```python
from build123d import *

# Parameters (mm, degrees)
ESQUISSE1_W                  = 70
ESQUISSE1_H                  = 25
BOSS_EXTRU_1_DEPTH           = 25
ENL_V_MAT_EXTRU_1_DEPTH      = 79.421935707
ENL_V_MAT_EXTRU_1_DEPTH_BACK = 79.421935707
CONG_1_R                     = 5
CONG_2_R                     = 2
ENL_V_MAT_EXTRU_2_DEPTH      = 79.421935739
ENL_V_MAT_EXTRU_2_DEPTH_BACK = 79.421935739
ESQUISSE3_R                  = 8


with BuildPart() as part:
    # Esquisse1 → Boss.-Extru.1 (new body)
    with BuildSketch(Plane.XY):
        with Locations((35, 12.5)):
            Rectangle(ESQUISSE1_W, ESQUISSE1_H)
    extrude(amount=BOSS_EXTRU_1_DEPTH)

    # Esquisse2 → Enlèv. mat.-Extru.1 (cut, two sides: drawn at the far end of the back side and taken through both)
    with BuildSketch(Plane.XY.offset(25).offset(-ENL_V_MAT_EXTRU_1_DEPTH_BACK)):
        with BuildLine():
            Line((30, 25), (0, 25))
            Line((0, 25), (0, 10))
            ThreePointArc((0, 10), (16.648162051, 14.203675898), (30, 25))
        make_face()
    extrude(amount=ENL_V_MAT_EXTRU_1_DEPTH + ENL_V_MAT_EXTRU_1_DEPTH_BACK, mode=Mode.SUBTRACT)

    # Congé1
    cong_1_edges = [part.edges().sort_by_distance(p)[0] for p in [
        (30, 25, 12.5),
        (0, 10, 12.5),
        (70, 25, 12.5),
        (70, 0, 12.5),
        (0, 0, 12.5),
    ]]
    fillet(cong_1_edges, radius=CONG_1_R)

    # Congé2
    cong_2_edges = [part.edges().sort_by_distance(p)[0] for p in [
        (35, 0, 0),
        (35, 0, 25),
        (17.598161914, 14.694657605, 0),
        (48.658916792, 25, 0),
        (70, 12.5, 0),
        (0, 5.207778491, 0),
        (68.535533906, 23.535533906, 0),
        (68.535533906, 1.464466094, 0),
        (1.227276928, 8.696800743, 0),
        (30.275283676, 24.563769261, 0),
        (1.464466094, 1.464466094, 0),
        (0, 5.207778491, 25),
        (48.658916792, 25, 25),
        (17.598161914, 14.694657605, 25),
        (70, 12.5, 25),
        (68.535533906, 23.535533906, 25),
        (68.535533906, 1.464466094, 25),
        (1.227276928, 8.696800743, 25),
        (30.275283676, 24.563769261, 25),
        (1.464466094, 1.464466094, 25),
    ]]
    fillet(cong_2_edges, radius=CONG_2_R)

    # Esquisse3 → Enlèv. mat.-Extru.2 (cut, two sides: drawn at the far end of the back side and taken through both)
    with BuildSketch(Plane(origin=(0, 25, 0), x_dir=(1, 0, 0), z_dir=(0, 1, 0)).offset(-ENL_V_MAT_EXTRU_2_DEPTH_BACK)):
        with Locations(Location((45, -12.5, 0), (0, 0, 270))):
            Circle(ESQUISSE3_R)
    extrude(amount=ENL_V_MAT_EXTRU_2_DEPTH + ENL_V_MAT_EXTRU_2_DEPTH_BACK, mode=Mode.SUBTRACT)


solid = part.part
```
Can you work these out from the model? Positions are in its coordinate system, mm. Give positions to 0.01 mm unless a question says otherwise; leave off trailing zeros. Order: outer loops, then holes, each group sorted by start corner. A loop starts at its lowest first (then second) coordinate and runs counter-clockwise, first axis right, second up. Notation, with made-up numbers: (31.25, 57) - (66.25, 57) arc R14 ccw to (66.25, 68) - close; hole circle Ø5 at (20, -19.75). An arc over 180 degrees is marked (long way). Use a Markdown table: item, result. Add a question column.
Q1. If we section it at B-B on x = 45: Write out the boundary of the cut face in (y, z), plus the area to 3 significant figures.
Q2. I'm going to push flat-ended pins straight in: pin 1 (8 mm diameter, centred on y = 21, z = 5, fed in from -X); pin 2 (13 mm diameter, centred on x = 45, z = 12.5, fed in from -Y); pin 3 (12 mm diameter, centred on y = 21.5, z = 7, fed in from -X). Where does each tip first touch, or does it pass through?
Q3. If we mould it in two halves opening along X, with no side actions, what happens to faces 1 (the cylindrical face through (52.932, 12.325, 11.459)), 2 (the flat face through (42, 10, 25)), 3 (the cylindrical face through (30.248, 24.552, 12.647)), 4 (the cylindrical face through (69.4, 12.6, 0.57))? For each: released by +X, released by -X, zero draft, split by the parting line, or undercut.
Q4. If we section it at C-C on z = 8.75: Write out the boundary of the cut face in (x, y).
Q5. If we section it at A-A on z = 12.5: Write out the boundary of the cut face in (x, y), plus the area to 3 significant figures.
Q6. Please list where these lines run through material, in increasing order: line 1 along Z through (x, y) = (45, 19.75); line 2 along X through (y, z) = (9, 16.25); line 3 along X through (y, z) = (18, 18.5).
Answers follow:
| question | item | result |
|---|---|---|
| 1 | outline | (0, 2) arc R2 ccw to (2, 0) - (23, 0) arc R2 ccw to (25, 2) - (25, 4.5) - (0, 4.5) - close; (0, 20.5) - (25, 20.5) - (25, 23) arc R2 ccw to (23, 25) - (2, 25) arc R2 ccw to (0, 23) - close |
| 1 | area | 222 mm^2 |
| 2 | pin 1 | stops at x = 21.39 |
| 2 | pin 2 | passes through |
| 2 | pin 3 | stops at x = 19.03 |
| 3 | face 1 | undercut |
| 3 | face 2 | zero draft |
| 3 | face 3 | released by -X |
| 3 | face 4 | released by +X |
| 4 | outline | (0, 5) arc R5 ccw to (5, 0) - (37.93, 0) - (37.93, 25) - (32.32, 25) arc R5 ccw to (28.59, 23.33) arc R40 cw to (4.31, 10.37) arc R5 ccw to (0, 5.42) - close; (52.07, 0) - (65, 0) arc R5 ccw to (70, 5) - (70, 20) arc R5 ccw to (65, 25) - (52.07, 25) - close |
| 5 | outline | (0, 5) arc R5 ccw to (5, 0) - (37, 0) - (37, 25) - (32.32, 25) arc R5 ccw to (28.59, 23.33) arc R40 cw to (4.31, 10.37) arc R5 ccw to (0, 5.42) - close; (53, 0) - (65, 0) arc R5 ccw to (70, 5) - (70, 20) arc R5 ccw to (65, 25) - (53, 25) - close |
| 5 | area | 1,020 mm^2 |
| 6 | line 1 | z = 0 to 4.5, 20.5 to 25 |
| 6 | line 2 | x = 1.51 to 37.93, 52.07 to 70 |
| 6 | line 3 | x = 22.79 to 39.71, 50.29 to 70 |
